Job drawing, mm, ordinate dimensions from the low corner. One solid piece. Round coordinates to 2 decimals unless told otherwise and drop trailing zeros. Order: outer loops, then holes, each group sorted by start corner. A loop starts at its lowest first (then second) coordinate and runs counter-clockwise, first axis right, second up. Notation, with made-up numbers: (47.25, -16) - (70.25, -16) arc R33 ccw to (70.25, 20) - close; hole circle Ø10 at (5, 78.5). An arc over 180 degrees is marked (long way). Use one line per item in the form item = value. Start each with the question number.
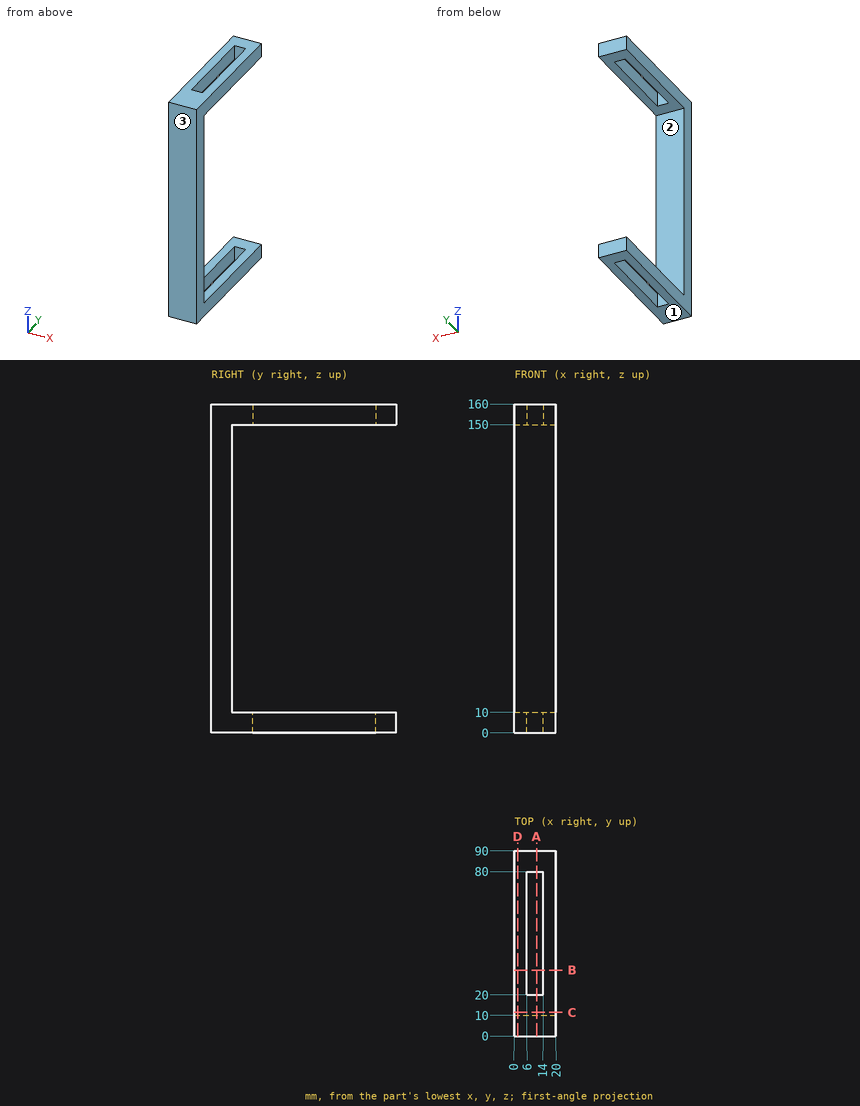
(1) Slice it at A-A (x = 10.75). Give the cut face in (y, z), and give its area (3 significant figures).
(2) Slice it at B-B (y = 32). Give the cut face in (x, z), and give its area (3 significant figures).
(3) Slice it at C-C (y = 11.5). Give the cut face in (x, z).
(4) Mould opens along Z. For the marked faces 1, 2 and 3 say: pulls with the +Z half, pulls with the -Z half, needs draft (parallel to the pull), parting line crosses it, or undercut.
(5) Slice it at D-D (x = 1.5). Give the cut face in (y, z).
(6) Wall check: line 1 (Z direction, x = 14.5, y = 17); line 2 (X direction, y = 47.5, z = 152); line 3 (Y direction, x = 18.75, z = 70.5). Give the ranges that are in metal, low to high. Write a range as [from, to].
(7) Flat gauge pins, fed straight in: P1, Ø2.5, axis at x = 8, z = 156.5, coming from the -Y side; P2, Ø1, axis at x = 8.5, z = 22.5, coming from the +Y side; P3, Ø6, axis at x = 9.5, y = 67.5, coming from the +Z side. Where does each tip first touch, or does it go through?
Results list:
q1.outline = (0, 0) - (20, 0) - (20, 10) - (10, 10) - (10, 150) - (20, 150) - (20, 160) - (0, 160) - close; (80, 0) - (90, 0) - (90, 10) - (80, 10) - close; (80, 150) - (90, 150) - (90, 160) - (80, 160) - close
q1.area = 2,000 mm²
q2.outline = (0, 0) - (6, 0) - (6, 10) - (0, 10) - close; (0, 150) - (6, 150) - (6, 160) - (0, 160) - close; (14, 0) - (20, 0) - (20, 10) - (14, 10) - close; (14, 150) - (20, 150) - (20, 160) - (14, 160) - close
q2.area = 240 mm²
q3.outline = (0, 0) - (20, 0) - (20, 10) - (0, 10) - close; (0, 150) - (20, 150) - (20, 160) - (0, 160) - close
q4.face_1 = pulls with the -Z half
q4.face_2 = undercut
q4.face_3 = needs draft
q5.outline = (0, 0) - (90, 0) - (90, 10) - (10, 10) - (10, 150) - (90, 150) - (90, 160) - (0, 160) - close
q6.line_1 = [0, 10], [150, 160]
q6.line_2 = [0, 6], [14, 20]
q6.line_3 = [0, 10]
q7.P1 = 0
q7.P2 = 10
q7.P3 = through
